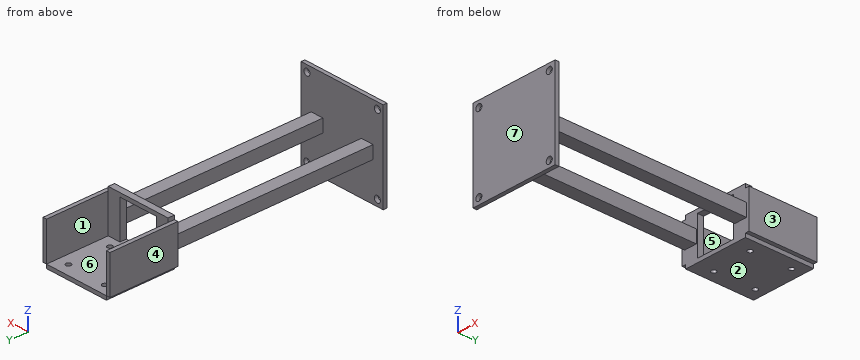
Autodesk Inventor part; units mm, degrees
ref_plane "YZ Plane" through (0, 0, 0) normal (1, 0, 0) x (0, 1, 0)
ref_plane "XZ Plane" through (0, 0, 0) normal (0, 1, 0) x (-1, 0, 0)
ref_plane "XY Plane" through (0, 0, 0) normal (0, 0, 1) x (1, 0, 0)
sketch "Boceto1" plane through (0, 0, 0) normal (0, 1, 0) x (-1, 0, 0)
  line L0 (25.5, 15) -> (-25.5, 15)
  line L1 (-25.5, 15) -> (-25.5, -15)
  line L2 (-25.5, -15) -> (25.5, -15)
  line L3 (25.5, -15) -> (25.5, 15)
  line L4 (25.5, 15) -> (-25.5, -15) construction
  line L5 (-25.5, 15) -> (25.5, -15) construction
  line L6 (-15.5, 15) -> (-15.5, -15)
  line L7 (0, 15) -> (0, 11.847)
  line L8 (-25.5, 0) -> (-22.3332, 0)
  line L9 (25.5, 15) -> (25.5, -15)
  line L10 (15.5, 15) -> (15.5, -15)
  line L11 (25.5, 0) -> (22.3332, 0)
  line L12 (-25.5, -15) -> (-25.5, 15)
  line L13 (-25.5, 0) -> (-22.3332, 0)
  line L14 (-25.5, 15) -> (-25.5, -15)
  point P0 (0, 0)
  point P1 (31.5, 22.5)
  dimension "d2" = 10
  dimension "d21" = 51
  dimension "d22" = 30
extrude "Extrusión1" add sketch "Boceto1" along normal blind 5 contours L3 L2 L10 L0 | L6 L2 L1 L0
sketch "Boceto4" plane through (0, 0, 0) normal (0, 1, 0) x (-1, 0, 0)
  line L0 (-28.5, 18) -> (28.5, 18)
  line L1 (28.5, 18) -> (28.5, -18)
  line L2 (28.5, -18) -> (-28.5, -18)
  line L3 (-28.5, -18) -> (-28.5, 18)
  line L4 (-28.5, 18) -> (28.5, -18) construction
  line L5 (28.5, 18) -> (-28.5, -18) construction
  line L6 (28.5, -15) -> (-28.5, -15)
  line L7 (-28.5, 15) -> (28.5, 15)
  line L8 (25.5, -18) -> (25.5, 18)
  line L9 (-25.5, 18) -> (-25.5, -18)
  line L10 (-25.5, -15) -> (-15.5, -15)
  point P0 (0, 0)
  point P1 (-25.5, -15)
  point P2 (-25.5, 15)
  point P3 (25.5, 15)
  point P4 (25.5, -15)
  dimension "d23" = 57
  dimension "d24" = 36
  dimension "d27" = 0
extrude "Extrusión4" add sketch "Boceto4" along normal blind 5 contours L0 L8 L7 L9 | L7 L9 L6 L3 | L7 L1 L6 L8 | L6 L8 L2 L9
sketch "Boceto5" plane through (0, 5, 0) normal (0, 1, 0) x (1, 0, 0)
  line L0 (25.5, 18) -> (-25.5, 18)
  line L1 (25.5, 15) -> (25.5, 18)
  line L2 (-25.5, 18) -> (25.5, 18)
  line L3 (25.5, 18) -> (25.5, 15)
  line L4 (25.5, 15) -> (-25.5, 15)
  line L5 (-25.5, 15) -> (-25.5, 18)
  point P0 (0, 0)
extrude "Extrusión5" add sketch "Boceto5" along normal blind 49
sketch "Boceto6" plane through (-15.5, 0, -15) normal (0, 0, 1) x (1, 0, 0)
  circle A0 centre (32, 45) radius 2
  line L0 (41, 5) -> (41, 54)
  line L1 (-10, 54) -> (41, 54)
  line L2 (-10, 5) -> (-10, 54)
  line L3 (-10, 29.5) -> (15.5, 29.5)
  line L4 (15.5, 29.5) -> (15.5, 54)
  circle A1 centre (0, 46) radius 2
  circle A2 centre (-1, 14) radius 2
  circle A3 centre (31, 13) radius 2
  point P0 (15.5, 0)
  dimension "d30" = 4
  dimension "d31" = 9
  dimension "d32" = 9
  dimension "d35" = 360
extrude "Extrusión6" cut sketch "Boceto6" against normal blind 49 contours A0 | A1 | A2 | A3
sketch "Boceto7" plane through (0, 5, 0) normal (0, 1, 0) x (1, 0, 0)
  line L0 (-28.5, 15) -> (-28.5, -15)
  line L1 (-28.5, 15) -> (-25.5, 15)
  line L2 (-25.5, 15) -> (-25.5, -15)
  line L3 (-25.5, -15) -> (-28.5, -15)
  line L4 (-28.5, -15) -> (-28.5, 15)
  line L5 (28.5, 15) -> (25.5, 15)
  line L6 (25.5, -15) -> (28.5, -15)
  line L7 (28.5, 15) -> (25.5, 15)
  line L8 (25.5, 15) -> (25.5, -15)
  line L9 (25.5, -15) -> (28.5, -15)
  line L10 (28.5, -15) -> (28.5, 15)
  point P0 (0, 0)
  point P1 (25.5, -18)
extrude "Extrusión7" add sketch "Boceto7" along normal blind 49
sketch "Boceto9" plane through (0, 0, 0) normal (0, -1, 0) x (1, 0, 0)
  line L0 (-15.5, 15) -> (-15.5, -15)
  line L1 (-25.5, 15) -> (-15.5, 15)
  line L2 (-15.5, 0) -> (-28.5, 0)
  line L3 (-28.5, -15) -> (-28.5, 15)
  line L4 (-26.3951, 5) -> (-16.3951, 5)
  line L5 (-16.3951, 5) -> (-16.3951, -5)
  line L6 (-16.3951, -5) -> (-26.3951, -5)
  line L7 (-26.3951, -5) -> (-26.3951, 5)
  line L8 (-26.3951, 5) -> (-16.3951, -5) construction
  line L9 (-16.3951, 5) -> (-26.3951, -5) construction
  line L10 (26.3951, -5) -> (16.3951, -5)
  line L11 (16.3951, -5) -> (16.3951, 5)
  line L12 (16.3951, 5) -> (26.3951, 5)
  line L13 (26.3951, 5) -> (26.3951, -5)
  line L14 (26.3951, -5) -> (16.3951, 5) construction
  line L15 (16.3951, -5) -> (26.3951, 5) construction
  point P0 (0, 0)
  point P1 (-21.3951, 0)
  point P2 (21.3951, 0)
  dimension "d41" = 10
  dimension "d42" = 10
  dimension "d45" = 360
extrude "Extrusión8" add sketch "Boceto9" along normal blind 160
sketch "Boceto11" plane through (0, -160, 0) normal (0, -1, 0) x (1, 0, 0)
  line L0 (-35, 35) -> (35, 35)
  line L1 (35, 35) -> (35, -35)
  line L2 (35, -35) -> (-35, -35)
  line L3 (-35, -35) -> (-35, 35)
  line L4 (-35, 35) -> (35, -35) construction
  line L5 (35, 35) -> (-35, -35) construction
  line L6 (-35, -35) -> (35, -35)
  line L7 (35, -35) -> (35, 35)
  line L8 (35, 35) -> (-35, 35)
  line L9 (-35, 35) -> (-35, -35)
  line L10 (-35, -35) -> (35, 35) construction
  line L11 (35, -35) -> (-35, 35) construction
  line L12 (30, 30) -> (-30, 30)
  line L13 (-30, 30) -> (-30, -30)
  line L14 (-30, -30) -> (30, -30)
  line L15 (30, -30) -> (30, 30)
  line L16 (30, 30) -> (-30, -30) construction
  line L17 (-30, 30) -> (30, -30) construction
  circle A0 centre (-30, 30) radius 2.6
  circle A1 centre (30, 30) radius 2.6
  circle A2 centre (30, -30) radius 2.6
  circle A3 centre (-30, -30) radius 2.6
  line L18 (-26.3951, 5) -> (-16.3951, 5)
  line L19 (-16.3951, 5) -> (-16.3951, -5)
  line L20 (-26.3951, 5) -> (-16.3951, 5)
  line L21 (-16.3951, 5) -> (-16.3951, -5)
  line L22 (-16.3951, -5) -> (-26.3951, -5)
  line L23 (-26.3951, -5) -> (-26.3951, 5)
  line L24 (16.3951, 5) -> (26.3951, 5)
  line L25 (26.3951, 5) -> (26.3951, -5)
  line L26 (16.3951, 5) -> (26.3951, 5)
  line L27 (26.3951, 5) -> (26.3951, -5)
  line L28 (26.3951, -5) -> (16.3951, -5)
  line L29 (16.3951, -5) -> (16.3951, 5)
  point P0 (0, 0)
  point P1 (0, 0)
  dimension "d52" = 70
  dimension "d53" = 70
  dimension "d54" = 70
  dimension "d55" = 70
  dimension "d56" = 60
  dimension "d57" = 5.2
  dimension "d58" = 5.2
  dimension "d59" = 5.2
  dimension "d60" = 5.2
extrude "Extrusión9" add sketch "Boceto11" against normal blind 3 contours L0 L1 L2 L3 | L12 A1 L15 A2 L14 A3 L13 A0
properties part number "depth-camera-base"
The listing builds one solid part. Answer for the finished solid, in the listing's coordinates (mm). Face numbers are marked on the shaded views. A direction names the side the tool comes from. Give positions to 0.01 mm unless a question says otherwise; leave off trailing zeros. Write each loop counter-clockwise with the first axis right and the second up, starting at its lowest first coordinate (ties: lowest second). Pieces come first, ordered by that corner, then holes. Notation, with made-up numbers: (77.25, 30) - (132.25, 30) arc R10 ccw to (132.25, 39) - close; hole circle Ø4 at (-15, 81). An arc over 180 degrees is marked (long way). Use one line per item in the form item = value. Start each with the question number.
1) A tool of negligible diameter and unlimited length cuts with its end or side. For the marked faces 1, 2 and 3, from which of +Z, -Z, +X, -X, +Y, -Y can it reach the whole face along a straight path? Write none if from no direction.
2) Find section A-A on z = -30. Determine the outline of the cut face in (x, y), plus the area to 3 significant figures.
3) The mould has two halves that part along X. Classify the marked faces 4, 5, 6 and 7: pulls with the +X half, pulls with the -X half, needs draft (parallel to the pull), parting line crosses it, or undercut.
4) Consider line 1 along X through (y, z) = (-158, 30); line 2 along Z through (x, y) = (17, -106.5). Determine where each line is inside the solid, lowest interval first. Write a range as from..to.
5) Find section C-C on x = 8.5. Determine the outline of the cut face in (y, z).
6) Flat-ended cylindrical pins translate along their axes: pin 1 Ø0.9 at (x, y) = (-26.5, 24.5) entering from -Z; pin 2 Ø3.5 at (x, y) = (27, 24) entering from -Z; pin 3 Ø4.5 at (x, z) = (-30, 30) entering from +Y; pin 4 Ø4 at (y, z) = (2.5, -3.5) entering from +X. Find the tip coordinate at first contact, or state that the pin passes through.
7) Find section B-B on y = -145.5. Determine the outline of the cut face in (x, z), plus the area to 3 significant figures.
8) Find section D-D on z = 1. Determine the outline of the cut face in (x, y), plus the area to 3 significant figures.
Geometry results:
q1.face_1 = +Z, +Y
q1.face_2 = -Z, +X, -X, +Y
q1.face_3 = +Z, -Z, +X, +Y
q2.outline = (-35, -160) - (-32.6, -160) - (-32.6, -157) - (-35, -157) - close; (-27.4, -160) - (27.4, -160) - (27.4, -157) - (-27.4, -157) - close; (32.6, -160) - (35, -160) - (35, -157) - (32.6, -157) - close
q2.area = 179 mm2
q3.face_4 = pulls with the -X half
q3.face_5 = undercut
q3.face_6 = undercut
q3.face_7 = needs draft
q4.line_1 = -35..-32.6, -27.4..27.4, 32.6..35
q4.line_2 = -5..5
q5.outline = (-160, -35) - (-157, -35) - (-157, 35) - (-160, 35) - close; (0, -18) - (54, -18) - (54, -15) - (0, -15) - close; (0, 15) - (5, 15) - (5, 18) - (0, 18) - close
q6.pin_1 = -15
q6.pin_2 = -18
q6.pin_3 = through
q6.pin_4 = 28.5
q7.outline = (-26.4, -5) - (-16.4, -5) - (-16.4, 5) - (-26.4, 5) - close; (16.4, -5) - (26.4, -5) - (26.4, 5) - (16.4, 5) - close
q7.area = 200 mm2
q8.outline = (-35, -160) - (35, -160) - (35, -157) - (26.4, -157) - (26.4, 0) - (28.5, 0) - (28.5, 54) - (25.5, 54) - (25.5, 5) - (15.5, 5) - (15.5, 0) - (16.4, 0) - (16.4, -157) - (-16.4, -157) - (-16.4, 0) - (-15.5, 0) - (-15.5, 5) - (-25.5, 5) - (-25.5, 54) - (-28.5, 54) - (-28.5, 0) - (-26.4, 0) - (-26.4, -157) - (-35, -157) - close
q8.area = 3,770 mm2
